from build123d import *

# Parameters (mm, degrees)
EXTRUDE_1_DEPTH      = 5
EXTRUDE_1_DEPTH_BACK = 5
SKETCH_2_R           = 1.2
CUT_EXTRUDE_1_DEPTH  = 6
SKETCH_3_R           = 1.2
CUT_EXTRUDE_2_DEPTH  = 6
FILLET_1_R           = 1
FILLET_2_R           = 5


with BuildPart() as part:
    # Sketch 1 → Extrude 1 (new body, two sides)
    with BuildSketch(Plane(origin=(0, 0, 0), x_dir=(0, 0, -1), z_dir=(1, 0, 0))) as extrude_1_sk:
        Polygon((0, 30), (0, 0), (30, 0), (30, 5), (5, 5), (5, 30), align=None)
    extrude(amount=EXTRUDE_1_DEPTH)
    extrude(extrude_1_sk.sketch, amount=-EXTRUDE_1_DEPTH_BACK)

    # Sketch 2 → Cut-Extrude 1 (cut, through all)
    with BuildSketch(Plane(origin=(0, 5, 0), x_dir=(1, 0, 0), z_dir=(0, 1, 0))):
        with Locations((0, 25)):
            Circle(SKETCH_2_R)
        with Locations((0, 15)):
            Circle(SKETCH_2_R)
    extrude(amount=-CUT_EXTRUDE_1_DEPTH, mode=Mode.SUBTRACT)

    # Sketch 3 → Cut-Extrude 2 (cut, through all)
    with BuildSketch(Plane(origin=(0, 0, -5), x_dir=(-1, 0, 0), z_dir=(0, 0, -1))):
        with Locations((0, 25)):
            Circle(SKETCH_3_R)
        with Locations((0, 15)):
            Circle(SKETCH_3_R)
    extrude(amount=-CUT_EXTRUDE_2_DEPTH, mode=Mode.SUBTRACT)

    # Fillet 1
    fillet_1_edges = [part.edges().sort_by_distance(p)[0] for p in [
        (-5, 2.5, -30),
        (5, 30, -2.5),
        (5, 2.5, -30),
        (-5, 30, -2.5),
    ]]
    fillet(fillet_1_edges, radius=FILLET_1_R)

    # Fillet 2
    fillet_2_edges = [part.edges().sort_by_distance(p)[0] for p in [
        (0, 5, -5),
        (0, 0, 0),
    ]]
    fillet(fillet_2_edges, radius=FILLET_2_R)


solid = part.part
Input: part model. Units: mm. Frame: model coordinates. A direction names the side the tool comes from. Give positions to 0.01 mm unless a question says otherwise; leave off trailing zeros. Loops run counter-clockwise (first coordinate to the right, second up) from the corner with the lowest first, then second, coordinate; pieces in that order, holes last. Notation, with made-up numbers: (81, -26.5) - (87, -26.5) arc R5 ccw to (87, -17.5) - close; hole circle Ø11 at (9, 14). An arc over 180 degrees is marked (long way). Use CSV: the item, a comma, the result in double quotes. Start each with the question number.
Item 1: Section C-C on x = 0. Return loops of the section in (y, z), then the cut area to 3 significant figures.
Item 2: Contact query for flat-ended pins moving along their axis: P1, Ø2, axis at x = 0, y = 25, coming from the -Z side; P2, Ø2, axis at x = -1, y = 23, coming from the -Z side; P3, Ø3, axis at x = -0.5, z = -23, coming from the +Y side. Output: stop coordinate, or through.
Item 3: Section D-D on x = -2.5. Return loops of the section in (y, z), then the cut area to 3 significant figures.
Item 4: Section A-A on z = -25. Return loops of the section in (x, y).
Item 5: Line query: line 1 (X direction, y = 3.9, z = -15); line 2 (Z direction, x = 0, y = 1.55); line 3 (Z direction, x = 0, y = 2.1). Output: solid intervals per line, ascending.
Item 6: Section B-B on y = 15. Return loops of the section in (x, z), then the cut area to 3 significant figures.
Item 7: Mould query, pull axis Y, two halves, no side actions, for faces 1 (the flat face through (5, 8, -5)), 2 (the cylindrical face through (-4.715, 29.699, -2.465)), 3 (the cylindrical face through (0.26, 23.83, -2.54)). Classes: pulls with the +Y half, pulls with the -Y half, needs draft (parallel to the pull), parting line crosses it, or undercut.
Item 8: Reachability of faces 4 (the flat face through (0, 20, -5)), 5 (the cylindrical face through (4.715, 2.535, -29.699)) from +Z, -Z, +X, -X, +Y, -Y: full face, straight path, thin tool, end or side. Return the list, or none.
Ans:
1,outline,"(0, -30) - (5, -30) - (5, -26.2) - (0, -26.2) - close; (0, -23.8) - (5, -23.8) - (5, -16.2) - (0, -16.2) - close; (0, -13.8) - (5, -13.8) - (5, -10) arc R5 cw to (10, -5) - (13.8, -5) - (13.8, 0) - (5, 0) arc R5 ccw to (0, -5) - close; (16.2, -5) - (23.8, -5) - (23.8, 0) - (16.2, 0) - close; (26.2, -5) - (30, -5) - (30, 0) - (26.2, 0) - close"
1,area,"227 mm2"
2,P1,"passes through"
2,P2,"stops at z = -5"
2,P3,"stops at y = 5"
3,outline,"(0, -30) - (5, -30) - (5, -10) arc R5 cw to (10, -5) - (30, -5) - (30, 0) - (5, 0) arc R5 ccw to (0, -5) - close"
3,area,"275 mm2"
4,outline,"(-5, 0) - (-1.2, 0) - (-1.2, 5) - (-5, 5) - close; (1.2, 0) - (5, 0) - (5, 5) - (1.2, 5) - close"
5,line 1,"x = -5 to -1.2, 1.2 to 5"
5,line 2,"z = -30 to -26.2, -23.8 to -16.2, -13.8 to -1.38"
5,line 3,"z = -30 to -26.2, -23.8 to -16.2, -13.8 to -0.93"
6,outline,"(-5, -5) - (-1.2, -5) - (-1.2, 0) - (-5, 0) - close; (1.2, -5) - (5, -5) - (5, 0) - (1.2, 0) - close"
6,area,"38.0 mm2"
7,face 1,"needs draft"
7,face 2,"pulls with the +Y half"
7,face 3,"undercut"
8,face 4,"-Z, +X, -X, +Y"
8,face 5,"-Z, +X, +Y, -Y"
